```python
from build123d import *

# Parameters (mm, degrees)
SKETCH1_R           = 20
SKETCH1_R_2         = 5
BOSS_EXTRUDE1_DEPTH = 7.5
SKETCH2_R           = 2.25
CUT_EXTRUDE1_DEPTH  = 12
CIRPATTERN1_COUNT   = 4
SKETCH3_R           = 2.25
CUT_EXTRUDE2_DEPTH  = 21
CIRPATTERN2_COUNT   = 2
CIRPATTERN2_ANGLE   = 90
SKETCH4_R           = 23.708466839
SKETCH4_R_2         = 10
CUT_EXTRUDE3_DEPTH  = 2
SKETCH5_R           = 10
SKETCH5_R_2         = 5
BOSS_EXTRUDE2_DEPTH = 5


with BuildPart() as part:
    # Sketch1 → Boss-Extrude1 (new body, symmetric)
    with BuildSketch(Plane(origin=(0, 0, 0), x_dir=(1, 0, 0), z_dir=(0, 1, 0))):
        Circle(SKETCH1_R)
        Circle(SKETCH1_R_2, mode=Mode.SUBTRACT)
    extrude(amount=BOSS_EXTRUDE1_DEPTH, both=True)

    # Sketch2 → Cut-Extrude1 (cut)
    with BuildSketch(Plane(origin=(0, 7.5, 0), x_dir=(1, 0, 0), z_dir=(0, 1, 0))):
        with Locations((-10.606601718, 10.606601718)):
            Circle(SKETCH2_R)
    cut_extrude1 = extrude(amount=-CUT_EXTRUDE1_DEPTH, mode=Mode.SUBTRACT)

    # CirPattern1: Cut-Extrude1 ×4 about axis
    cirpattern1_axis = Axis((0, 0, 0), (0, 1, 0))
    for i in range(1, CIRPATTERN1_COUNT):
        add(cut_extrude1.rotate(cirpattern1_axis, i * 360 / CIRPATTERN1_COUNT), mode=Mode.SUBTRACT)

    # Sketch3 → Cut-Extrude2 (cut, through all)
    with BuildSketch(Plane.XY):
        Circle(SKETCH3_R)
    cut_extrude2 = extrude(amount=-CUT_EXTRUDE2_DEPTH, mode=Mode.SUBTRACT)

    # CirPattern2: Cut-Extrude2 ×2 about axis
    cirpattern2_axis = Axis((0, 7.5, 0), (0, 1, 0))
    for i in range(1, CIRPATTERN2_COUNT):
        add(cut_extrude2.rotate(cirpattern2_axis, i * CIRPATTERN2_ANGLE / (CIRPATTERN2_COUNT - 1)), mode=Mode.SUBTRACT)

    # Sketch4 → Cut-Extrude3 (cut)
    with BuildSketch(Plane.XZ.offset(7.5)):
        Circle(SKETCH4_R)
        Circle(SKETCH4_R_2, mode=Mode.SUBTRACT)
    extrude(amount=-CUT_EXTRUDE3_DEPTH, mode=Mode.SUBTRACT)

    # Sketch5 → Boss-Extrude2 (add)
    with BuildSketch(Plane(origin=(0, 7.5, 0), x_dir=(1, 0, 0), z_dir=(0, 1, 0))):
        Circle(SKETCH5_R)
        Circle(SKETCH5_R_2, mode=Mode.SUBTRACT)
    extrude(amount=BOSS_EXTRUDE2_DEPTH)


solid = part.part
```
Verification items for the finished model (mm, model axes). A direction names the side the tool comes from. Give positions to 0.01 mm unless a question says otherwise; leave off trailing zeros. Order: outer loops, then holes, each group sorted by start corner. A loop starts at its lowest first (then second) coordinate and runs counter-clockwise, first axis right, second up. Notation, with made-up numbers: M 1.5,7 L 36.5,7 A21 cw 36.5,28 Z; hole C -21.75,-20.75 d7. An arc over 180 degrees is marked long. Answer in a Markdown table with one row per item. Add a question column.
Item 1: Section check B-B, the plane z = 0. Enter the section's corners in (x, y).
Item 2: Section check D-D, the plane x = -9.5. Enter the section's corners in (y, z).
Item 3: Section check A-A, the plane x = 0. Enter the section's corners in (y, z), and give its area (4 significant figures).
Item 4: Mould release check, pull along X, two halves, no side actions. Record for faces 1 (the flat face through (-5, 7.5, -9)), 2 (the cylindrical face through (-12.504, 1.584, 9.397)), 3 (the cylindrical face through (18.475, 1.091, 7.66)): released by +X, released by -X, zero draft, split by the parting line, or undercut.
Item 5: Tool access check on faces 4 (the cylindrical face through (-12.12, 2.23, 0.29)), 5 (the cylindrical face through (-2.17, 9.96, 9.76)), 6 (the flat face through (2, -7.5, -5)), 7 (the cylindrical face through (-2.17, -6.51, -9.76)), 8 (the cylindrical face through (-0.29, 2.23, -12.13)). Record the directions out of +Z, -Z, +X, -X, +Y, -Y that give a thin tool (end or side, any length) a straight path to the whole face; none if there is none.
Item 6: Gauge pin test, flat ends, axial feed: pin 1 (2.5 mm diameter, centred on x = -10.61, z = -10.61, fed in from -Y); pin 2 (2 mm diameter, centred on x = 11.5, z = -11, fed in from +Y); pin 3 (16 mm diameter, centred on x = 0, z = 0, fed in from -Y); pin 4 (4 mm diameter, centred on y = -3, z = -11, fed in from -X). Record the tip position at first contact, or that the pin passes through.
Item 7: Scan lines: probe 1 along X at (y, z) = (4.5, 0); probe 2 along X at (y, z) = (11.5, 0); probe 3 along X at (y, z) = (-3, 11). Record each from-to range of solid material in increasing order. Write a range as from..to.
Item 8: Section check C-C, the plane y = -1. Enter the section's corners in (x, z).
Filled sheet:
| question | item | result |
|---|---|---|
| 1 | outline | M -20,-5.5 L -10,-5.5 L -10,-7.5 L -5,-7.5 L -5,-2.25 L -20,-2.25 Z; M -20,2.25 L -5,2.25 L -5,12.5 L -10,12.5 L -10,7.5 L -20,7.5 Z; M 5,-7.5 L 10,-7.5 L 10,-5.5 L 20,-5.5 L 20,7.5 L 10,7.5 L 10,12.5 L 5,12.5 Z |
| 2 | outline | M -7.5,-3.12 L -5.5,-3.12 L -5.5,-17.6 L 7.5,-17.6 L 7.5,-12.57 L -4.5,-12.57 L -4.5,-8.65 L 7.5,-8.65 L 7.5,-3.12 L 12.5,-3.12 L 12.5,3.12 L 7.5,3.12 L 7.5,8.65 L -4.5,8.65 L -4.5,12.57 L 7.5,12.57 L 7.5,17.6 L -5.5,17.6 L -5.5,3.12 L -7.5,3.12 Z; hole C 0,0 d4.5 |
| 3 | outline | M -7.5,-10 L -5.5,-10 L -5.5,-20 L -2.25,-20 L -2.25,-5 L -7.5,-5 Z; M -7.5,5 L 12.5,5 L 12.5,10 L 7.5,10 L 7.5,20 L -5.5,20 L -5.5,10 L -7.5,10 Z; M 2.25,-20 L 7.5,-20 L 7.5,-10 L 12.5,-10 L 12.5,-5 L 2.25,-5 Z |
| 3 | area | 392.5 mm^2 |
| 4 | face 1 | zero draft |
| 4 | face 2 | undercut |
| 4 | face 3 | split by the parting line |
| 5 | face 4 | -X |
| 5 | face 5 | +Y |
| 5 | face 6 | +Z, -Z, +X, -X, -Y |
| 5 | face 7 | -Y |
| 5 | face 8 | -Z |
| 6 | pin 1 | stops at y = -5.5 |
| 6 | pin 2 | stops at y = -4.5 |
| 6 | pin 3 | stops at y = -7.5 |
| 6 | pin 4 | stops at x = -17.86 |
| 7 | probe 1 | x = -20..-5, 5..20 |
| 7 | probe 2 | x = -10..-5, 5..10 |
| 7 | probe 3 | x = -16.7..-12.82, -8.39..8.39, 12.82..16.7 |
| 8 | outline | M -19.9,-2.02 A20 ccw -2.02,-19.9 L -2.02,-4.58 A5 cw -4.58,-2.02 Z; M -19.9,2.02 L -4.58,2.02 A5 cw long 2.02,-4.58 L 2.02,-19.9 A20 ccw long Z; hole C -10.61,-10.61 d4.5; hole C -10.61,10.61 d4.5; hole C 10.61,-10.61 d4.5; hole C 10.61,10.61 d4.5 |
